Could you check a few things on this model? Use its own coordinates, in mm. A direction names the side the tool comes from. Coordinates: 2 decimals unless noted, no trailing zeros. Loops run counter-clockwise (first coordinate to the right, second up) from the corner with the lowest first, then second, coordinate; pieces in that order, holes last. Notation, with made-up numbers: (15, 35.25) - (40, 35.25) arc R4 ccw to (40, 39.25) - close; hole circle Ø6 at (68, 55). An arc over 180 degrees is marked (long way). Put each result on its own line as item: value. Start each with the question number.
```python
from build123d import *

# Parameters (mm, degrees)
F0_W     = 20
F0_H     = 20
F1_DEPTH = 20
F2_R     = 2.5
F3_DEPTH = 2.5
F4_R     = 2.5
F5_DEPTH = 2.5
F7_DEPTH = 2.5
F8_R     = 2
F9_DEPTH = 6


with BuildPart() as f1:
    # F0 (on Front) → F1 (new body)
    with BuildSketch(Plane.XZ):
        with Locations((-28.577724, 9.489656)):
            Rectangle(F0_W, F0_H)
    extrude(amount=F1_DEPTH)

    # F2 (on face) → F3 (cut)
    with BuildSketch(Plane.XZ.offset(20)):
        with Locations((-33.577724, 14.489656)):
            Circle(F2_R)
    extrude(amount=-F3_DEPTH, mode=Mode.SUBTRACT)

    # F4 (on face) → F5 (cut)
    with BuildSketch(Plane.XZ.offset(20)):
        with Locations((-23.577724, 14.489656)):
            Circle(F4_R)
    extrude(amount=-F5_DEPTH, mode=Mode.SUBTRACT)

    # F6 (on face) → F7 (cut)
    with BuildSketch(Plane.XZ.offset(20)):
        Polygon((-34.428626, 7.275801), (-35.029531, 6.263753), (-33.796098, 3.955018), (-32.878928, 5.37821), (-31.898506, 3.923391), (-30.918086, 5.536343), (-30.095795, 3.955018), (-29.33676, 5.56797), (-28.103326, 3.923391), (-27.470795, 5.726102), (-26.363868, 3.765259), (-25.130434, 6.706524), (-25.573205, 7.275801), align=None)
    extrude(amount=-F7_DEPTH, mode=Mode.SUBTRACT)

    # F8 (on face) → F9 (cut)
    with BuildSketch(Plane.YZ.offset(-18.577724)):
        with Locations((-10.681243, 9.938739)):
            Circle(F8_R)
    extrude(amount=-F9_DEPTH, mode=Mode.SUBTRACT)


solid = f1.part
```
(1) If we mould it in two halves opening along X, with no side actions, what happens to faces 4 (the flat face through (-24.578, -11, 10)), 5 (the flat face through (-29, 0, 10)), 6 (the flat face through (-32.396, -18.768, 4.661))? For each: pulls with the +X half, pulls with the -X half, needs draft (parallel to the pull), parting line crosses it, or undercut.
(2) Which directions (+Z, -Z, +X, -X, +Y, -Y) give clear straight access to the entire face, cutting with the end or side of a thin tool? Please do faces 1 (the flat face through (-38.578, -10, 9)), 2 (the cylindrical face through (-21.536, -12.155, 11.29)), 3 (the flat face through (-34.421, -18.768, 5.126)).
(3) I want a section at D-D on z = 15. List the corners of the cut face in (x, y) for me.
(4) For pin 1 Ø2 at (y, z) = (-10.5, 10) entering from +X, with a flat end and sliding along its axis, tell me the tip position at first contact or that it passes through.
(5) I want a section at C-C on y = -9. List the corners of the cut face in (x, z) for me, and give its area (3 significant figures).
(6) I need wall thicknesses on L1, parallel to Z at x = -29.75, y = -19; L2, parallel to Y at x = -23, z = 8.25; L3, parallel to Z at x = -22.5, y = -18.75. Which ranges of each line are inside material? Lowest first, please. Write a range as [from, to].
(7) I want a section at A-A on z = 8.75. List the corners of the cut face in (x, y) for me, and give its area (3 significant figures).
(8) I want a section at B-B on x = -22.5. List the corners of the cut face in (y, z) for me.
Answer sheet:
1. face 4: pulls with the +X half
1. face 5: needs draft
1. face 6: undercut
2. face 1: +Z, -Z, -X, +Y, -Y
2. face 2: +X
2. face 3: -Y
3. outline: (-38.58, -20) - (-36.03, -20) - (-36.03, -17.5) - (-31.13, -17.5) - (-31.13, -20) - (-26.03, -20) - (-26.03, -17.5) - (-21.13, -17.5) - (-21.13, -20) - (-18.58, -20) - (-18.58, 0) - (-38.58, 0) - close
4. pin 1: stops at x = -24.58
5. outline: (-38.58, -0.51) - (-18.58, -0.51) - (-18.58, 8.86) - (-24.58, 8.86) - (-24.58, 11.02) - (-18.58, 11.02) - (-18.58, 19.49) - (-38.58, 19.49) - close
5. area: 387 mm^2
6. L1: z = [-0.51, 4.69], [7.28, 19.49]
6. L2: y = [-20, -11.75], [-9.61, 0]
6. L3: z = [-0.51, 12.23], [16.75, 19.49]
7. outline: (-38.58, -20) - (-18.58, -20) - (-18.58, -12.29) - (-24.58, -12.29) - (-24.58, -9.07) - (-18.58, -9.07) - (-18.58, 0) - (-38.58, 0) - close
7. area: 381 mm^2
8. outline: (-20, -0.51) - (0, -0.51) - (0, 19.49) - (-20, 19.49) - (-20, 16.75) - (-17.5, 16.75) - (-17.5, 12.23) - (-20, 12.23) - close; hole circle Ø4 at (-10.68, 9.94)
